Geometry: final body of the model. Coordinates: model frame, mm. Round coordinates to 2 decimals unless told otherwise and drop trailing zeros. Write each loop counter-clockwise with the first axis right and the second up, starting at its lowest first coordinate (ties: lowest second). Pieces come first, ordered by that corner, then holes. Notation, with made-up numbers: (68.25, -11.75) - (92.25, -11.75) arc R17 ccw to (92.25, -6.75) - close; hole circle Ø5 at (61.5, 43). An arc over 180 degrees is marked (long way). Write each question's results on one line, items separated by ' | '.
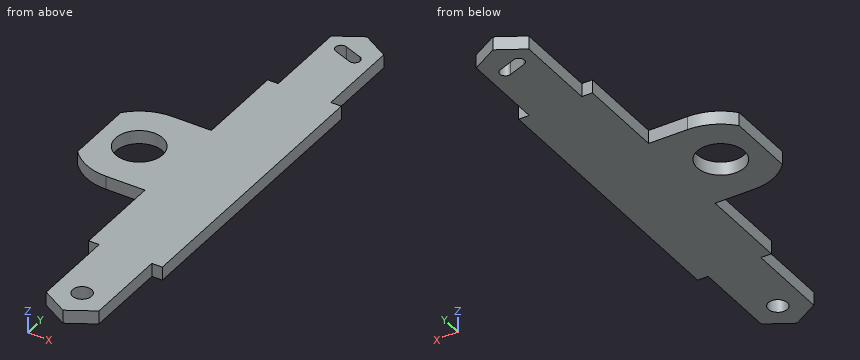
Autodesk Inventor part; units mm, degrees
ref_plane "YZ Plane" through (0, 0, 0) normal (1, 0, 0) x (0, 1, 0)
ref_plane "XZ Plane" through (0, 0, 0) normal (0, 1, 0) x (-1, 0, 0)
ref_plane "XY Plane" through (0, 0, 0) normal (0, 0, 1) x (1, 0, 0)
sketch "Sketch1" plane through (0, 0, 0) normal (0, 0, 1) x (1, 0, 0)
  line L0 (12.5, -107.2169) -> (-12.5, -107.2169)
  line L1 (-12.5, -107.2169) -> (-12.5, 107.2169)
  line L2 (-12.5, 107.2169) -> (12.5, 107.2169)
  line L3 (12.5, 107.2169) -> (12.5, -107.2169)
  line L4 (12.5, -107.2169) -> (-12.5, 107.2169) construction
  line L5 (-12.5, -107.2169) -> (12.5, 107.2169) construction
  line L6 (0, 100) -> (0, -100) construction
  line L7 (-12.5, 107.2169) -> (0, 114.4338)
  line L8 (0, 114.4338) -> (12.5, 107.2169)
  line L9 (12.5, 107.2169) -> (12.5, 92.7831)
  line L10 (12.5, 92.7831) -> (0, 85.5662)
  line L11 (0, 85.5662) -> (-12.5, 92.7831)
  line L12 (-12.5, 92.7831) -> (-12.5, 107.2169)
  line L13 (-12.5, -107.2169) -> (-12.5, -92.7831)
  line L14 (-12.5, -92.7831) -> (0, -85.5662)
  line L15 (0, -85.5662) -> (12.5, -92.7831)
  line L16 (12.5, -92.7831) -> (12.5, -107.2169)
  line L17 (12.5, -107.2169) -> (0, -114.4338)
  line L18 (0, -114.4338) -> (-12.5, -107.2169)
  line L19 (-4.2122, 101.5835) -> (4.2122, 98.4165) construction
  line L20 (-5.1447, 99.103) -> (3.2797, 95.936)
  line L21 (5.1447, 100.897) -> (-3.2797, 104.064)
  arc A0 (-3.2797, 104.064) -> (-5.1447, 99.103) centre (-4.2122, 101.5835) ccw
  arc A1 (3.2797, 95.936) -> (5.1447, 100.897) centre (4.2122, 98.4165) ccw
  circle A2 centre (0, -100) radius 4.5
  circle A3 centre (-36, 0) radius 11.2
  circle A4 centre (-36, 0) radius 21 construction
  line L22 (-21, -14.6969) -> (-51, -14.6969) construction
  line L23 (-51, -14.6969) -> (-51, 14.6969) construction
  line L24 (-51, 14.6969) -> (-21, 14.6969) construction
  line L25 (-21, 14.6969) -> (-21, -14.6969) construction
  line L26 (-21, -14.6969) -> (-51, 14.6969) construction
  line L27 (-51, -14.6969) -> (-21, 14.6969) construction
  circle A5 centre (-36, 0) radius 25
  line L28 (-55, 16.2481) -> (-55, -16.2481)
  line L29 (-12.5, 25) -> (-36, 25)
  line L30 (-36, 25) -> (-36, -25)
  line L31 (-36, -25) -> (-12.5, -25)
  line L32 (-12.5, -25) -> (-12.5, 25)
  line L33 (17.5, -67.375) -> (-17.5, -67.375)
  line L34 (-17.5, -67.375) -> (-17.5, 67.375)
  line L35 (-17.5, 67.375) -> (17.5, 67.375)
  line L36 (17.5, 67.375) -> (17.5, -67.375)
  line L37 (17.5, -67.375) -> (-17.5, 67.375) construction
  line L38 (-17.5, -67.375) -> (17.5, 67.375) construction
  point P0 (0, 0)
  point P1 (266, 0)
  point P2 (-17.5, -25)
  point P3 (-12.5, -67.375)
  point P4 (-12.5, 67.375)
  point P5 (-17.5, 25)
  point P6 (-36, 25)
  point P7 (12.5, 67.375)
  point P8 (12.5, -67.375)
  dimension "d8" = 42
  dimension "d0" = 25
  dimension "d1" = 266
  dimension "d2" = 200
  dimension "d3" = 5.3
  dimension "d4" = 9
  dimension "d5" = 9
  dimension "d6" = 22.4
  dimension "d7" = 36
  dimension "d9" = 30
  dimension "d10" = 4
  dimension "d11" = 4
  dimension "d12" = 134.75
  dimension "d13" = 35
extrude "Extrusion1" add sketch "Sketch1" along normal blind 6.35 contours L17 L18 L0 | L0 L1 L14 L15 L3 | L15 L14 L1 L33 L3 | L33 L1 A5 L35 L3 | L3 L35 L36 L33 | L33 L34 L31 L1 | L35 L1 L11 L10 L3 | L31 L34 A5 L1 | L10 L11 L1 L2 L3 | L1 L29 L34 L35 | A5 L34 L1 | L1 A5 | L31 A5 L34 | L2 L7 L8 | L1 A5 L34 L29 | A5 L30 A3 L34 | A5 L28 L30 A3 | L34 A5 L29
sketch "Sketch2" plane through (0, 0, 6.35) normal (0, 0, 1) x (1, 0, 0)
  line L0 (-17.5, -25) -> (-17.5, -67.375)
  line L1 (-17.5, -67.375) -> (-12.5, -67.375)
  line L2 (-12.5, -67.375) -> (-12.5, -107.2169)
  line L3 (-12.5, -107.2169) -> (0, -114.4338)
  line L4 (0, -114.4338) -> (12.5, -107.2169)
  line L5 (12.5, -107.2169) -> (12.5, -67.375)
  line L6 (12.5, -67.375) -> (17.5, -67.375)
  line L7 (17.5, -67.375) -> (17.5, 67.375)
  line L8 (17.5, 67.375) -> (12.5, 67.375)
  line L9 (12.5, 67.375) -> (12.5, 107.2169)
  line L10 (12.5, 107.2169) -> (0, 114.4338)
  line L11 (0, 114.4338) -> (-12.5, 107.2169)
  line L12 (-12.5, 107.2169) -> (-12.5, 67.375)
  line L13 (-12.5, 67.375) -> (-17.5, 67.375)
  line L14 (-17.5, 67.375) -> (-17.5, 25)
  line L15 (-17.5, 25) -> (-36, 25)
  arc A0 (-36, 25) -> (-55, 16.2481) centre (-36, 0) ccw
  line L16 (-55, 16.2481) -> (-55, -16.2481)
  arc A1 (-55, -16.2481) -> (-36, -25) centre (-36, 0) ccw
  line L17 (-36, -25) -> (-17.5, -25)
  circle A2 centre (-36, 0) radius 11.2
  arc A3 (-3.2797, 104.064) -> (-5.1447, 99.103) centre (-4.2122, 101.5835) ccw
  line L18 (-3.2797, 104.064) -> (5.1447, 100.897)
  arc A4 (3.2797, 95.936) -> (5.1447, 100.897) centre (4.2122, 98.4165) ccw
  line L19 (3.2797, 95.936) -> (-5.1447, 99.103)
  circle A5 centre (0, -100) radius 4.5
  circle A6 centre (-13.25, 68.125) radius 1.375
  point P0 (0, 0)
  point P1 (-12.5, 69.2774)
  point P2 (-14.4024, 67.375)
  dimension "d16" = 0.75
  dimension "d17" = 2.75
  dimension "d18" = 0.75
sketch "Sketch3" plane through (0, 0, 6.35) normal (0, 0, 1) x (1, 0, 0)
  circle A0 centre (0, -100) radius 4.5
  arc A1 (-3.2797, 104.064) -> (-5.1447, 99.103) centre (-4.2122, 101.5835) ccw
  line L0 (-3.2797, 104.064) -> (5.1447, 100.897)
  arc A2 (3.2797, 95.936) -> (5.1447, 100.897) centre (4.2122, 98.4165) ccw
  line L1 (3.2797, 95.936) -> (-5.1447, 99.103)
  circle A3 centre (-36, 0) radius 11.2
  arc A4 (14.4024, -67.375) -> (12.5, -69.2774) centre (13.25, -68.125) ccw
  line L2 (14.4024, -67.375) -> (17.5, -67.375)
  line L3 (17.5, -67.375) -> (17.5, 67.375)
  line L4 (17.5, 67.375) -> (14.4024, 67.375)
  arc A5 (12.5, 69.2774) -> (14.4024, 67.375) centre (13.25, 68.125) ccw
  line L5 (12.5, 69.2774) -> (12.5, 107.2169)
  line L6 (12.5, 107.2169) -> (0, 114.4338)
  line L7 (0, 114.4338) -> (-12.5, 107.2169)
  line L8 (-12.5, 107.2169) -> (-12.5, 69.2774)
  arc A6 (-14.4024, 67.375) -> (-12.5, 69.2774) centre (-13.25, 68.125) ccw
  line L9 (-14.4024, 67.375) -> (-17.5, 67.375)
  line L10 (-17.5, 67.375) -> (-17.5, 25)
  line L11 (-17.5, 25) -> (-36, 25)
  arc A7 (-36, 25) -> (-55, 16.2481) centre (-36, 0) ccw
  line L12 (-55, 16.2481) -> (-55, -16.2481)
  arc A8 (-55, -16.2481) -> (-36, -25) centre (-36, 0) ccw
  line L13 (-36, -25) -> (-17.5, -25)
  line L14 (-17.5, -25) -> (-17.5, -67.375)
  line L15 (-17.5, -67.375) -> (-14.4024, -67.375)
  arc A9 (-12.5, -69.2774) -> (-14.4024, -67.375) centre (-13.25, -68.125) ccw
  line L16 (-12.5, -69.2774) -> (-12.5, -107.2169)
  line L17 (-12.5, -107.2169) -> (0, -114.4338)
  line L18 (0, -114.4338) -> (12.5, -107.2169)
  line L19 (12.5, -107.2169) -> (12.5, -69.2774)
  circle A10 centre (-36, 0) radius 16 construction
  line L20 (-36, 0) -> (-24.6863, 11.3137) construction
  line L21 (-36, 0) -> (-36, 16) construction
  line L22 (-36, 0) -> (-36, -16) construction
  line L23 (-47.3137, -11.3137) -> (-24.6863, -11.3137) construction
  line L24 (-24.6863, -11.3137) -> (-24.6863, 11.3137) construction
  line L25 (-24.6863, 11.3137) -> (-47.3137, 11.3137) construction
  line L26 (-47.3137, 11.3137) -> (-47.3137, -11.3137) construction
  line L27 (-47.3137, -11.3137) -> (-24.6863, 11.3137) construction
  line L28 (-24.6863, -11.3137) -> (-47.3137, 11.3137) construction
  point P0 (0, 0)
  dimension "d21" = 32
  dimension "d22" = 45
sketch "Sketch4" plane through (0, 0, 6.35) normal (0, 0, 1) x (1, 0, 0)
  line L0 (10, -57.375) -> (-10, -57.375) construction
  line L1 (-10, -57.375) -> (-10, 57.375) construction
  line L2 (-10, 57.375) -> (10, 57.375) construction
  line L3 (10, 57.375) -> (10, -57.375) construction
  line L4 (10, -57.375) -> (-10, 57.375) construction
  line L5 (-10, -57.375) -> (10, 57.375) construction
  line L6 (-17.5, -67.375) -> (-14.4024, -67.375) construction
  point P0 (0, 0)
  point P1 (-10, 0)
  point P2 (10, 0)
  dimension "d30" = 20
  dimension "d32" = 10
equation "\"d11\" = d10"
equation "\"d18\" = d16"
properties part number "Z-Axis Nut and Bed Plate" material "Aluminum 6061"
Q1. Ray query, line 1 along Y through (x, z) = (-3, 0.75); line 2 along X through (y, z) = (0, 2); line 3 along Y through (x, z) = (-36, 4). Return the intervals inside material, ascending.
Answer block:
line 1: -112.7 to -103.35, -96.65 to 98.3, 103.96 to 112.7 | line 2: -55 to -47.2, -24.8 to 17.5 | line 3: -25 to -11.2, 11.2 to 25
Q2. Section query B-B, the plane x = -38. Return loops of the section in (y, z), plus the area to 3 significant figures.
Answer block:
outline: (-24.92, 0) - (-11.02, 0) - (-11.02, 6.35) - (-24.92, 6.35) - close; (11.02, 0) - (24.92, 0) - (24.92, 6.35) - (11.02, 6.35) - close | area: 177 mm2
Q3. Section query D-D, the plane x = -22.5. Return loops of the section in (y, z), plus the area to 4 significant figures.
Answer block:
outline: (-25, 0) - (25, 0) - (25, 6.35) - (-25, 6.35) - close | area: 317.5 mm2
Q4. Pin query (flat end, axial travel): pin 1 (2.5 mm diameter, centred on x = -16, z = 3, fed in from -Y) (3 decimals); pin 2 (3 mm diameter, centred on y = 63.5, z = 4.5, fed in from -X); pin 3 (1.5 mm diameter, centred on x = 14.5, z = 4.5, fed in from +Y) (3 decimals). Return the tip coordinate at first contact, or that it passes through.
Answer block:
pin 1: y = -67.375 | pin 2: x = -17.5 | pin 3: y = 67.375
Q5. Section query C-C, the plane z = 3.5. Return loops of the section in (x, y) (1 decimal).
Answer block:
outline: (-55, -16.2) arc R25 ccw to (-36, -25) - (-17.5, -25) - (-17.5, -67.4) - (-12.5, -67.4) - (-12.5, -107.2) - (0, -114.4) - (12.5, -107.2) - (12.5, -67.4) - (17.5, -67.4) - (17.5, 67.4) - (12.5, 67.4) - (12.5, 107.2) - (0, 114.4) - (-12.5, 107.2) - (-12.5, 67.4) - (-17.5, 67.4) - (-17.5, 25) - (-36, 25) arc R25 ccw to (-55, 16.2) - close; hole circle Ø22.4 at (-36, 0); hole (-5.1, 99.1) - (3.3, 95.9) arc R2.6 ccw to (5.1, 100.9) - (-3.3, 104.1) arc R2.6 ccw to start; hole circle Ø9 at (0, -100)
Q6. Section query A-A, the plane y = 0. Return loops of the section in (x, z), plus the area to 3 significant figures.
Answer block:
outline: (-55, 0) - (-47.2, 0) - (-47.2, 6.35) - (-55, 6.35) - close; (-24.8, 0) - (17.5, 0) - (17.5, 6.35) - (-24.8, 6.35) - close | area: 318 mm2
